Autodesk Inventor part; units mm, degrees
ref_plane "工作平面1" through (0, -10, 0) normal (0, 1, 0) x (-1, 0, 0)
ref_plane "工作平面2" through (0, 0, 162.2) normal (0, 0, -1) x (-1, 0, 0)
ref_plane "YZ Plane" through (0, 0, 0) normal (1, 0, 0) x (0, 1, 0)
sketch "草图1" plane through (0, 0, 0) normal (0, 0, 1) x (1, 0, 0)
  circle A0 centre (0, 0) radius 10
  dimension "d0" = 20
extrude "拉伸1" add sketch "草图1" along normal blind 237.2
ref_plane "工作平面1" through (0, -10, 0) normal (0, 1, 0) x (-1, 0, 0)
sketch "草图2" plane through (0, -10, 0) normal (0, 1, 0) x (-1, 0, 0)
  line L0 (3, 33.7) -> (-3, 33.7)
  line L1 (-3, 33.7) -> (-3, 11.7)
  line L2 (-3, 11.7) -> (3, 11.7)
  line L3 (3, 11.7) -> (3, 33.7)
  arc A0 (3, 33.7) -> (-3, 33.7) centre (0, 33.7) ccw
  arc A1 (-3, 11.7) -> (3, 11.7) centre (0, 11.7) ccw
  line L4 (0, 0) -> (0, 11.7)
  dimension "d3" = 6
  dimension "d4" = 22
  dimension "d5" = 11.7
extrude "拉伸2" cut sketch "草图2" along normal blind 2.5
sketch "草图3" plane through (0, 0, 0) normal (0, 1, 0) x (-1, 0, 0)
  line L0 (-9.175, 5.2) -> (-16.1829, 5.2)
  line L1 (-16.1829, 5.2) -> (-16.1829, 4)
  line L2 (-16.1829, 4) -> (-9.175, 4)
  line L3 (-9.175, 4) -> (-9.175, 5.2)
  line L4 (0, 0) -> (0, -12.502)
  line L5 (-10, 0) -> (10, 0)
  dimension "d8" = 12.502
  dimension "d9" = 4
  dimension "d10" = 1.2
  dimension "d11" = 9.175
  dimension "d12" = 7.0079
revolve "旋转1" cut sketch "草图3" angle 360 about axis through (0, 0, 0) along (0, 0, -1)
chamfer "倒角1" distance 0.5 angle 45 1 edges at (-10, 0, 0)
ref_plane "工作平面2" through (0, 0, 162.2) normal (0, 0, -1) x (-1, 0, 0)
sketch "草图4" plane through (0, 0, 162.2) normal (0, 0, -1) x (-1, 0, 0)
  circle A0 centre (0, 0) radius 12
  circle A1 centre (0, 0) radius 10
  dimension "d18" = 24
extrude "拉伸3" add sketch "草图4" against normal blind 10
chamfer "倒角2" distance 0.5 angle 45 1 edges at (-10, 0, 237.2)
sketch "草图5" plane through (0, 0, 0) normal (0, 1, 0) x (-1, 0, 0)
  line L0 (-12, 234.9) -> (-9.175, 234.9)
  line L1 (-9.175, 234.9) -> (-9.175, 233.7)
  line L2 (-9.175, 233.7) -> (-12, 233.7)
  line L3 (-12, 233.7) -> (-12, 234.9)
  line L4 (-9.5, 237.2) -> (9.5, 237.2)
  line L5 (10, 236.7) -> (-10, 236.7)
  line L6 (0, 236.7) -> (0, 240.4719)
  point P0 (0, 0)
  dimension "d24" = 1.2
  dimension "d25" = 2.3
  dimension "d26" = 3.7719
  dimension "d27" = 12
  dimension "d29" = 9.175
revolve "旋转2" cut sketch "草图5" angle 360 about axis through (0, 0, 236.7) along (0, 0, 1)
properties part number "齿轮60-2万向轴"
Check sheet for the modelled part. Datum: model origin and axes. Units: mm. A direction names the side the tool comes from. Give positions to 0.01 mm unless a question says otherwise; leave off trailing zeros. Write each loop counter-clockwise with the first axis right and the second up, starting at its lowest first coordinate (ties: lowest second). Pieces come first, ordered by that corner, then holes.
Item 1: Scan lines: L1, parallel to Y at x = -3.25, z = 110; L2, parallel to Z at x = -9.5, y = -4.75; L3, parallel to Y at x = 0.75, z = 108. Record each from-to range of solid material in increasing order.
Item 2: Gauge pin test, flat ends, axial feed: pin 1 (1 mm diameter, centred on x = 1.5, z = 57, fed in from -Y); pin 2 (8 mm diameter, centred on y = -7.5, z = 108.5, fed in from +X); pin 3 (3 mm diameter, centred on x = -0.5, z = 24.5, fed in from -Y); pin 4 (1 mm diameter, centred on x = 3, y = 6, fed in from -Z). Record the tip position at first contact, or that the pin passes through.
Item 3: Access from +Z, -Z, +X, -X, +Y, -Y to the whole of each face (thin tool, end or side, straight path). Record for faces 5 (the face through (0, -7.5, 23)), 6 (the face through (9, 3, 4)), 7 (the face through (-2.17, 9.76, 235.79)), 8 (the face through (5, 9, 162.2)).
Item 4: Draft check along Z on faces 1 (the face through (0, 0, 0)), 2 (the face through (-2.17, 9.76, 2.23)), 3 (the face through (8.75, -2.76, 234.29)), 4 (the face through (5, 9, 172.2)). Enter one of: released by +Z, released by -Z, zero draft, split by the parting line, or undercut.
Item 5: Cross-section at B-B (z = 118). Enter the section's corners in (x, y), and give its area (3 significant figures).
Report:
1. L1: y = -9.46 to 9.46
1. L2: z = 162.2 to 172.2
1. L3: y = -9.97 to 9.97
2. pin 1: stops at y = -9.95
2. pin 2: stops at x = 9.37
2. pin 3: stops at y = -7.5
2. pin 4: stops at z = 0
3. face 5: -Y
3. face 6: none
3. face 7: +Z
3. face 8: -Z
4. face 1: released by -Z
4. face 2: zero draft
4. face 3: undercut
4. face 4: released by +Z
5. outline: circle Ø20 at (0, 0)
5. area: 314 mm2
